from build123d import *

# Parameters (mm, degrees)
BOSS_EXTRUDE1_DEPTH = 20
SKETCH2_R           = 1.75
CUT_EXTRUDE1_DEPTH  = 13
FILLET1_R           = 1


with BuildPart() as part:
    # Sketch1 → Boss-Extrude1 (new body)
    with BuildSketch(Plane(origin=(0, 0, 0), x_dir=(1, 0, 0), z_dir=(0, 1, 0))):
        with BuildLine():
            Line((-18, 0), (-18, -12))
            Line((-18, -12), (18, -12))
            Line((18, -12), (18, 0))
            Line((18, 0), (9.987492178, 0))
            ThreePointArc((9.987492178, 0), (0, -9.5), (-9.987492178, 0))
            Line((-9.987492178, 0), (-18, 0))
        make_face()
    extrude(amount=BOSS_EXTRUDE1_DEPTH)

    # Sketch2 → Cut-Extrude1 (cut, through all)
    with BuildSketch(Plane.XY.offset(12)):
        with Locations((-14, 16)):
            Circle(SKETCH2_R)
        with Locations((-14, 4)):
            Circle(SKETCH2_R)
        with Locations((14, 4)):
            Circle(SKETCH2_R)
        with Locations((14, 16)):
            Circle(SKETCH2_R)
    extrude(amount=-CUT_EXTRUDE1_DEPTH, mode=Mode.SUBTRACT)

    # Fillet1
    fillet1_edges = [part.edges().sort_by_distance(p)[0] for p in [
        (-18, 20, 6),
        (-18, 0, 6),
        (18, 0, 6),
        (18, 20, 6),
    ]]
    fillet(fillet1_edges, radius=FILLET1_R)


solid = part.part
Source: CAD feature listing. Evaluate the final solid. Frame: model axes, mm. Round coordinates to 2 decimals unless told otherwise and drop trailing zeros. Loops run counter-clockwise (first coordinate to the right, second up) from the corner with the lowest first, then second, coordinate; pieces in that order, holes last. Notation, with made-up numbers: M 23,-27.75 L 68,-27.75 A23 ccw 68,-12.75 Z; hole C 64.5,78.5 d9. An arc over 180 degrees is marked long. Return JSON: item names as keys, results as strings. Group by question number.
1. Material intervals for line 1 along Y through (x, z) = (-14, 8.25); line 2 along X through (y, z) = (14.5, 11.5); line 3 along X through (y, z) = (2.5, 1.5), sorted ascending. Write a range as from..to.
2. Section query C-C on z = 7.25. Output: boundary loops of the cut face in (x, y), and give its area (3 significant figures).
3. Section query A-A on y = 16. Output: boundary loops of the cut face in (x, z), and give its area (3 significant figures).
4. Mould query, pull axis Y, two halves, no side actions, for faces 1 (the face through (14.81, 2.45, 6.08)), 2 (the face through (-17.715, 19.699, 6.084)), 3 (the face through (14, 10, 0)). Classes: released by +Y, released by -Y, zero draft, split by the parting line, or undercut.
5. Section query D-D on z = 10.5. Output: boundary loops of the cut face in (x, y), and give its area (3 significant figures).
6. Section query B-B on x = 14. Output: boundary loops of the cut face in (y, z), and give its area (3 significant figures).
7. Pin query (flat end, axial travel): pin 1 (1 mm diameter, centred on x = -1, y = 6, fed in from -Z). Return the tip coordinate at first contact, or that it passes through.
Checks:
{
 "1": {"line 1": "y = 0..2.25, 5.75..14.25, 17.75..20", "line 2": "x = -18..-14.9, -13.1..13.1, 14.9..18", "line 3": "x = -18..-14.9, -13.1..-9.8, 9.8..13.1, 14.9..18"},
 "2": {"outline": "M -18,1 A1 ccw -17,0 L -6.32,0 L -6.32,20 L -17,20 A1 ccw -18,19 Z; M 6.32,0 L 17,0 A1 ccw 18,1 L 18,19 A1 ccw 17,20 L 6.32,20 Z; hole C -14,4 d3.5; hole C -14,16 d3.5; hole C 14,4 d3.5; hole C 14,16 d3.5", "area": "428 mm²"},
 "3": {"outline": "M -18,0 L -15.75,0 L -15.75,12 L -18,12 Z; M -12.25,0 L -9.99,0 A10 cw 9.99,0 L 12.25,0 L 12.25,12 L -12.25,12 Z; M 15.75,0 L 18,0 L 18,12 L 15.75,12 Z", "area": "201 mm²"},
 "4": {"face 1": "undercut", "face 2": "released by +Y", "face 3": "zero draft"},
 "5": {"outline": "M -18,1 A1 ccw -17,0 L 17,0 A1 ccw 18,1 L 18,19 A1 ccw 17,20 L -17,20 A1 ccw -18,19 Z; hole C -14,4 d3.5; hole C -14,16 d3.5; hole C 14,4 d3.5; hole C 14,16 d3.5", "area": "681 mm²"},
 "6": {"outline": "M 0,0 L 2.25,0 L 2.25,12 L 0,12 Z; M 5.75,0 L 14.25,0 L 14.25,12 L 5.75,12 Z; M 17.75,0 L 20,0 L 20,12 L 17.75,12 Z", "area": "156 mm²"},
 "7": {"pin 1": "stops at z = 9.39"}
}
